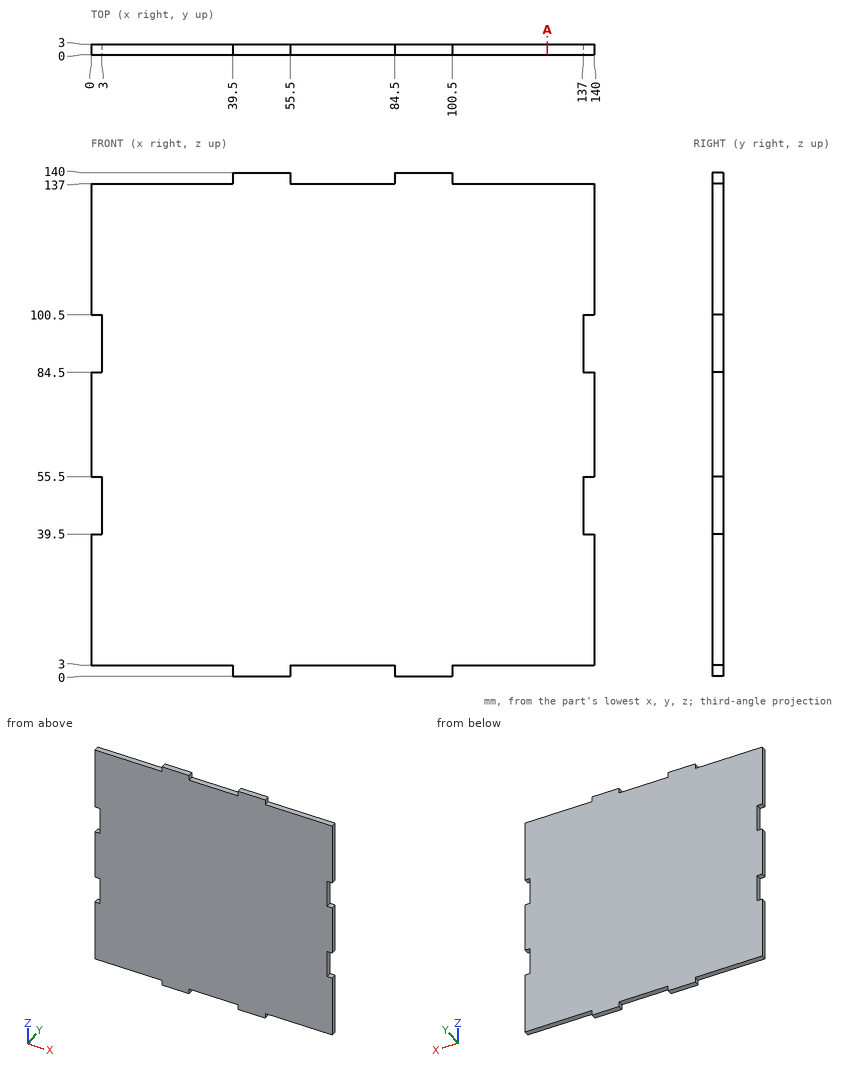
Geometry: see drawing. Coordinates: mm, zero at the bounding-box minimum. Give positions to 0.01 mm unless a question says otherwise; leave off trailing zeros. Order: outer loops, then holes, each group sorted by start corner. A loop starts at its lowest first (then second) coordinate and runs counter-clockwise, first axis right, second up. Notation, with made-up numbers: M 32,-4.75 L 44,-4.75 A22 ccw 44,16.25 Z; hole C -9.5,86.5 d8. An arc over 180 degrees is marked long. Answer as a JSON object with one key per item and string values.
1. First-contact query: P1, Ø0.9, axis at y = 1, z = 48.5, coming from the -X side; P2, Ø0.9, axis at y = 1.5, z = 138, coming from the +X side; P3, Ø0.9, axis at x = 2, y = 1.5, coming from the -Z side. Flat tips, straight axial feed; report the tip coordinate or a pass-through.
Result sheet:
{"P1": "x = 3", "P2": "x = 100.5", "P3": "z = 3"}
2. Ray query, line 1 (Z direction, x = 78.5, y = 2.8). Return the intervals inside material, ascending. Write a range as [from, to].
Result sheet:
{"line 1": "[3, 137]"}
3. Cut plane A-A, the plane x = 127. Output: boundary loops of the cut face in (y, z).
Result sheet:
{"outline": "M 0,3 L 3,3 L 3,137 L 0,137 Z"}
